Work out the finished part from the listing and answer in its coordinate system (mm). Face numbers are marked on the shaded views. A direction names the side the tool comes from. Round coordinates to 2 decimals unless told otherwise and drop trailing zeros. Loops run counter-clockwise (first coordinate to the right, second up) from the corner with the lowest first, then second, coordinate; pieces in that order, holes last. Notation, with made-up numbers: (42, -32) - (88, -32) arc R8 cw to (88, -22) - close; hole circle Ø3 at (4.5, 89). An arc over 180 degrees is marked (long way). Answer as CSV lines item,"result". Start each with the question number.
```python
from build123d import *

# Parameters (mm, degrees)
F0_W      = 609.6
F0_H      = 457.2
F1_DEPTH  = 76.2
F3_DEPTH  = 76.201
F5_D      = 8
F6_W      = 127
F6_H      = 203.2
F7_DEPTH  = 25.4
F9_DEPTH  = 76.201
F11_DEPTH = 25.4
F12_R     = 9.525
F14_D     = 7.9375
F16_D     = 7.9375
F16_DEPTH = 12.7
F16_TIP   = 2.3846655818


# Not quite as in the source:
# - a feature names something its author has since deleted; it is built from what else it names


with BuildPart() as f1:
    # F0 (on Top) → F1 (new body)
    with BuildSketch(Plane.XY):
        with Locations((304.8, -228.6)):
            Rectangle(F0_W, F0_H)
    extrude(amount=-F1_DEPTH)

    # F2 (on Top) → F3 (cut, through all)
    with BuildSketch(Plane.XY):
        Polygon((392.35, -89.85), (367.35, -64.85), (109.35, -64.85), (84.35, -89.85), (84.35, -369.85), (112.35, -391.85), (364.35, -391.85), (392.35, -369.85), align=None)
    extrude(amount=-F3_DEPTH, mode=Mode.SUBTRACT)

    # F5 (through all)
    with Locations(Plane.XY):
        with Locations((69.35, -67.85), (389.35, -67.85), (389.35, -387.85), (69.35, -304.85)):
            Hole(F5_D / 2)

    # F6 (on Top) → F7 (cut)
    with BuildSketch(Plane.XY):
        with Locations((479.525, -127)):
            Rectangle(F6_W, F6_H)
    extrude(amount=-F7_DEPTH, mode=Mode.SUBTRACT)

    # F8 (on Top) → F9 (cut, through all)
    with BuildSketch(Plane.XY):
        Polygon((454.125, -25.4), (416.025, -63.5), (416.025, -190.5), (454.125, -228.6), (504.925, -228.6), (543.025, -190.5), (543.025, -63.5), (504.925, -25.4), align=None)
    extrude(amount=-F9_DEPTH, mode=Mode.SUBTRACT)

    # F10 (on face) → F11 (cut)
    with BuildSketch(Plane(origin=(0, 0, -76.2), x_dir=(1, 0, 0), z_dir=(0, 0, -1))):
        Polygon((398.875, 25.4), (416.025, 25.4), (543.025, 25.4), (543.025, 228.6), (416.025, 228.6), (398.875, 228.6), (398.875, 397.375), (59.825, 397.375), (59.825, 58.325), (398.875, 58.325), align=None)
    extrude(amount=-F11_DEPTH, mode=Mode.SUBTRACT)

    # F12
    f12_edges = [f1.edges().sort_by_distance(p)[0] for p in [
        (364.35, -391.85, -25.4),
        (392.35, -369.85, -25.4),
        (392.35, -89.85, -25.4),
        (367.35, -64.85, -25.4),
        (109.35, -64.85, -25.4),
        (84.35, -89.85, -25.4),
        (84.35, -369.85, -25.4),
        (112.35, -391.85, -25.4),
        (59.825, -397.375, -63.5),
        (59.825, -58.325, -63.5),
        (398.875, -58.325, -63.5),
        (398.875, -25.4, -63.5),
        (543.025, -25.4, -63.5),
        (543.025, -228.6, -63.5),
        (398.875, -228.6, -63.5),
        (398.875, -397.375, -63.5),
        (454.125, -228.6, -38.1),
        (416.025, -190.5, -38.1),
        (504.925, -228.6, -38.1),
        (543.025, -190.5, -38.1),
        (416.025, -63.5, -38.1),
        (454.125, -25.4, -38.1),
        (504.925, -25.4, -38.1),
        (543.025, -63.5, -38.1),
        (416.025, -25.4, -12.7),
        (543.025, -25.4, -12.7),
        (416.025, -228.6, -12.7),
        (543.025, -228.6, -12.7),
    ]]
    fillet(f12_edges, radius=F12_R)

    # F14 (through all)
    with Locations(Plane.XY):
        with Locations((427.1375, -36.5125), (531.9125, -36.5125), (531.9125, -217.4875), (427.1375, -217.4875)):
            Hole(F14_D / 2)

    # F16
    with Locations(Plane(origin=(0, 0, -76.2), x_dir=(1, 0, 0), z_dir=(0, 0, -1))):
        with Locations((34.925, 422.275), (574.675, 422.275), (574.675, 34.925), (34.925, 34.925)):
            Hole(F16_D / 2, depth=F16_DEPTH)
            with Locations((0, 0, -(F16_DEPTH + F16_TIP / 2))):  # 118° drill point
                Cone(0, F16_D / 2, F16_TIP, mode=Mode.SUBTRACT)


solid = f1.part
```
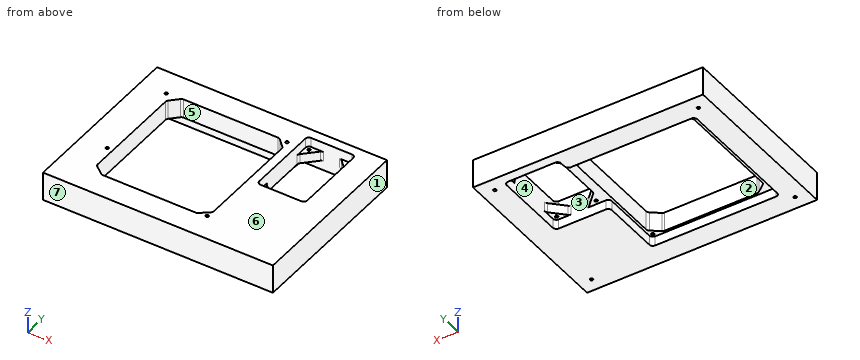
Item 1: Flat-ended cylindrical pins translate along their axes: pin 1 Ø5 at (x, y) = (574.675, -34.925) entering from -Z; pin 2 Ø12.5 at (x, y) = (524.5, -206.5) entering from -Z; pin 3 Ø7 at (x, y) = (531.91, -36.51) entering from +Z. Find the tip coordinate at first contact, or state that the pin passes through.
Item 2: Section B-B, the plane x = 207 is taken. Give the vertices of the cut face in (y, z) (3 decimals).
Item 3: Which of the six approach directions +Z, -Z, +X, -X, +Y, -Y give full straight-line access (tool end or side, diameter ignored) to the marked faces 1, 2 and 3?
Item 4: Find the intervals of material crossed by L1, parallel to X at y = -182, z = -28 (3 decimals); L2, parallel to X at y = -304, z = -26; L3, parallel to Y at x = 176, z = -63.5 (3 decimals), in increasing order.
Item 5: Section C-C, the plane x = 516 is taken. Give the vertices of the cut face in (y, z) (3 decimals), and give its area (3 significant figures).
Item 6: Determine the mould class of the marked faces 4, 5, 6 and 7 for opening direction Y: pulls with the +Y half, pulls with the -Y half, needs draft (parallel to the pull), parting line crosses it, or undercut.
Item 7: Section D-D, the plane z = -35 is taken. Count the separate pieces of the cut face and the enclosed holes in it, and give its area (3 significant figures).
Item 8: Section A-A, the plane y = -332 is taken. Give the vertices of the cut face in (x, z) (3 decimals).
Answer:
1,pin 1,"stops at z = -62.62"
1,pin 2,"stops at z = -50.8"
1,pin 3,"passes through"
2,outline,"(-457.2, -76.2) - (-397.375, -76.2) - (-397.375, -50.8) - (-391.85, -50.8) - (-391.85, 0) - (-457.2, 0) - close; (-64.85, -50.8) - (-58.325, -50.8) - (-58.325, -76.2) - (0, -76.2) - (0, 0) - (-64.85, 0) - close"
3,face 1,"+Z, -Z, +X, +Y, -Y"
3,face 2,"+Z, -Z"
3,face 3,"none"
4,L1,"x = 0 to 84.35, 392.35 to 416.025, 543.025 to 609.6"
4,L2,"x = 0 to 65.44, 73.26 to 84.35, 392.35 to 609.6"
4,L3,"y = -457.2 to -397.375, -58.325 to 0"
5,outline,"(-457.2, -76.2) - (-228.6, -76.2) - (-228.6, -50.8) - (-217.525, -50.8) - (-217.525, -25.4) - (-228.6, -25.4) - (-228.6, 0) - (-457.2, 0) - close; (-36.475, -50.8) - (-25.4, -50.8) - (-25.4, -76.2) - (0, -76.2) - (0, 0) - (-25.4, 0) - (-25.4, -25.4) - (-36.475, -25.4) - close"
5,area,"19,900 mm²"
6,face 4,"undercut"
6,face 5,"undercut"
6,face 6,"needs draft"
6,face 7,"pulls with the -Y half"
7,separate pieces,"1"
7,enclosed holes,"10"
7,area,"156,000 mm²"
8,outline,"(0, -76.2) - (59.825, -76.2) - (59.825, -50.8) - (84.35, -50.8) - (84.35, 0) - (0, 0) - close; (392.35, -50.8) - (398.875, -50.8) - (398.875, -76.2) - (609.6, -76.2) - (609.6, 0) - (392.35, 0) - close"
